from build123d import *

# Parameters (mm, degrees)
BOSS_EXTRUDE1_DEPTH      = 1.5875
BOSS_EXTRUDE1_DEPTH_BACK = 1.5875
SKETCH1_W                = 135
SKETCH1_H                = 60
CUT_EXTRUDE1_DEPTH       = 74.883490417
CUT_EXTRUDE1_DEPTH_BACK  = 74.883490417
SKETCH2_R                = 2.6
CUT_EXTRUDE2_DEPTH       = 74.883490417
LPATTERN1_COUNT          = 8
LPATTERN1_PITCH          = 15


with BuildPart() as part:
    # Sketch1 → Boss-Extrude1 (new, two sides: drawn at the far end of the back side and taken through both)
    with BuildSketch(Plane(origin=(0, 0, 0), x_dir=(0, 0, -1), z_dir=(1, 0, 0)).offset(-BOSS_EXTRUDE1_DEPTH_BACK)):
        Rectangle(SKETCH1_W, SKETCH1_H)
    extrude(amount=BOSS_EXTRUDE1_DEPTH + BOSS_EXTRUDE1_DEPTH_BACK)

    # Sketch2 → Cut-Extrude1 (cut, two sides: drawn at the far end of the back side and taken through both)
    with BuildSketch(Plane(origin=(0, 0, 0), x_dir=(0, 0, -1), z_dir=(1, 0, 0)).offset(-CUT_EXTRUDE1_DEPTH_BACK)):
        with Locations((-61.05, 23.55)):
            Circle(SKETCH2_R)
        with Locations(Location((61.05, 23.55, 0), (0, 0, 180))):
            Circle(SKETCH2_R)
        with Locations((61.05, -23.55)):
            Circle(SKETCH2_R)
        with Locations(Location((-61.05, -23.55, 0), (0, 0, 180))):
            Circle(SKETCH2_R)
    extrude(amount=CUT_EXTRUDE1_DEPTH + CUT_EXTRUDE1_DEPTH_BACK, mode=Mode.SUBTRACT)

    # Sketch3 → Cut-Extrude2 (cut, symmetric)
    with BuildSketch(Plane(origin=(0, 0, 0), x_dir=(0, 0, -1), z_dir=(1, 0, 0))):
        with BuildLine():
            Line((-56.6, -2.398436991), (-56.6, 2.398436991))
            ThreePointArc((-56.6, 2.398436991), (-52.5, 4.75), (-48.4, 2.398436991))
            Line((-48.4, 2.398436991), (-48.4, -2.398436991))
            ThreePointArc((-48.4, -2.398436991), (-52.5, -4.75), (-56.6, -2.398436991))
        make_face()
    cut_extrude2 = extrude(amount=CUT_EXTRUDE2_DEPTH, both=True, mode=Mode.SUBTRACT)

    # LPattern1: Cut-Extrude2 ×8
    with Locations(*[(0, 0, -i * LPATTERN1_PITCH) for i in range(1, LPATTERN1_COUNT)]):
        add(cut_extrude2, mode=Mode.SUBTRACT)


solid = part.part
Input: part model. Units: mm. Frame: model coordinates. A direction names the side the tool comes from. Give positions to 0.01 mm unless a question says otherwise; leave off trailing zeros. Write each loop counter-clockwise with the first axis right and the second up, starting at its lowest first coordinate (ties: lowest second). Pieces come first, ordered by that corner, then holes.
Q1. Section D-D, the plane x = 0.9. State how many separate pieces and enclosed holes the cut face has, plus the area to 3 significant figures.
Q2. Section B-B, the plane z = 61.05. Output: boundary loops of the cut face in (x, y).
Q3. Set-up query: faces 1 (the face through (0, 0, -67.5)), 2 (the face through (0.02, 4.75, -37.43)). Return all of +Z, -Z, +X, -X, +Y, -Y with unobstructed straight access to the full face (end or side cutting, diameter ignored); none if empty.
Q4. Section C-C, the plane y = 23.55. Output: boundary loops of the cut face in (x, z), plus the area to 3 significant figures.
Q5. Material intervals for probe 1 along Y at (x, z) = (-0.6, 61.05); probe 2 along Y at (x, z) = (-0.3, -22); probe 3 along Z at (x, y) = (1.3, 22.5), sorted ascending.
Q6. First-contact query: P1, Ø3, axis at y = 23.55, z = -61.05, coming from the -X side; P2, Ø6, axis at y = 23.55, z = 61.05, coming from the +X side. Flat tips, straight axial feed; report the tip coordinate or a pass-through.
Q7. Pull-direction query (Y, two-part tool) for faces 3 (the face through (1.588, 0, 1)), 4 (the face through (0.02, -4.75, -22.57)); classes: pulls with the +Y half, pulls with the -Y half, needs draft (parallel to the pull), parting line crosses it, or undercut.
Q8. Section A-A, the plane z = -52.5. Output: boundary loops of the cut face in (x, y).
Filled in:
1. separate pieces: 1
1. enclosed holes: 12
1. area: 7,480 mm2
2. outline: (-1.59, -30) - (1.59, -30) - (1.59, -26.15) - (-1.59, -26.15) - close; (-1.59, -20.95) - (1.59, -20.95) - (1.59, 20.95) - (-1.59, 20.95) - close; (-1.59, 26.15) - (1.59, 26.15) - (1.59, 30) - (-1.59, 30) - close
3. face 1: -Z, +X, -X, +Y, -Y
3. face 2: +X, -X
4. outline: (-1.59, -67.5) - (1.59, -67.5) - (1.59, -63.65) - (-1.59, -63.65) - close; (-1.59, -58.45) - (1.59, -58.45) - (1.59, 58.45) - (-1.59, 58.45) - close; (-1.59, 63.65) - (1.59, 63.65) - (1.59, 67.5) - (-1.59, 67.5) - close
4. area: 396 mm2
5. probe 1: y = -30 to -26.15, -20.95 to 20.95, 26.15 to 30
5. probe 2: y = -30 to -4.72, 4.72 to 30
5. probe 3: z = -67.5 to -63.43, -58.67 to 58.67, 63.43 to 67.5
6. P1: passes through
6. P2: stops at x = 1.59
7. face 3: needs draft
7. face 4: undercut
8. outline: (-1.59, -30) - (1.59, -30) - (1.59, -4.75) - (-1.59, -4.75) - close; (-1.59, 4.75) - (1.59, 4.75) - (1.59, 30) - (-1.59, 30) - close
